Model file for the job. Use its own axes, mm. A direction names the side the tool comes from. Give positions to 0.01 mm unless a question says otherwise; leave off trailing zeros. Order: outer loops, then holes, each group sorted by start corner. A loop starts at its lowest first (then second) coordinate and runs counter-clockwise, first axis right, second up. Notation, with made-up numbers: M 35,-6.75 L 64,-6.75 A27 cw 64,30.25 Z; hole C 86.5,80.5 d1. An arc over 180 degrees is marked long. Return JSON: item names as keys, results as strings. Group by question number.
1. 3-axis set-ups, long thin cutter, end or side, ignore diameter. For faces 1 (the face through (38, 56, 3)), 2 (the face through (25.03, 56.1, 2.54)): which of +Z, -Z, +X, -X, +Y, -Y reach the whole face in a straight line?
2. Slice it at A-A on x = 29. List the corners of the cut face in (y, z), then the cut area to 3 significant figures.
3. Wall check: probe 1 along Y at (x, z) = (59, 1.3); probe 2 along Y at (x, z) = (9, 3); probe 3 along Y at (x, z) = (26, 0.9). Give the ranges that are in metal, low to high. Write a range as [from, to].
4. Pin check, flat tips, straight feed: pin 1 (1 mm diameter, centred on x = 39, z = 2, fed in from +Y); pin 2 (1 mm diameter, centred on y = 39, z = 2, fed in from +X); pin 3 (8 mm diameter, centred on x = 59.14, y = 29, fed in from -Z); pin 4 (2 mm diameter, centred on y = 56, z = 2, fed in from +X). Stop position of each tip, or through.
5. Slice it at D-D on z = 3.2. List the corners of the cut face in (x, y).
6. Slice it at B-B on x = 61.5. List the corners of the cut face in (y, z), then the cut area to 3 significant figures.
from build123d import *

# Parameters (mm, degrees)
BOSS_EXTRU_1_DEPTH      = 5
ESQUISSE3_W             = 38
ESQUISSE3_H             = 14
ESQUISSE3_W_2           = 14
ESQUISSE3_H_2           = 38
BOSS_EXTRU_2_DEPTH      = 5
ESQUISSE4_R             = 5
ESQUISSE4_R_2           = 3.5
ENL_V_MAT_EXTRU_2_DEPTH = 97.497156926
CONG_1_R                = 10


with BuildPart() as part:
    # Esquisse1 → Boss.-Extru.1 (new body)
    with BuildSketch(Plane.XY):
        Polygon((0, 0), (54.142135624, 0), (54.142135624, 40), (40, 54.142135624), (0, 54.142135624), align=None)
    extrude(amount=BOSS_EXTRU_1_DEPTH)

    # Esquisse3 → Boss.-Extru.2 (add)
    with BuildSketch(Plane.XY.offset(5)):
        with Locations((19, 61.142135624)):
            Rectangle(ESQUISSE3_W, ESQUISSE3_H)
        with Locations((61.142135624, 19)):
            Rectangle(ESQUISSE3_W_2, ESQUISSE3_H_2)
    extrude(amount=-BOSS_EXTRU_2_DEPTH)

    # Esquisse4 → Enlèv. mat.-Extru.2 (cut, through all)
    with BuildSketch(Plane.XY.offset(5)):
        with Locations((29, 59.142135624)):
            Circle(ESQUISSE4_R)
        with Locations(Location((9, 59.142135624, 0), (0, 0, 180))):
            Circle(ESQUISSE4_R)
        with Locations((59.142135624, 9)):
            Circle(ESQUISSE4_R)
        with Locations(Location((59.142135624, 29, 0), (0, 0, 180))):
            Circle(ESQUISSE4_R)
        with Locations((9.899494937, 9.899494937)):
            Circle(ESQUISSE4_R_2)
    extrude(amount=-ENL_V_MAT_EXTRU_2_DEPTH, mode=Mode.SUBTRACT)

    # Congé1
    cong_1_edges = [part.edges().sort_by_distance(p)[0] for p in [
        (0, 68.142135624, 2.5),
        (38, 68.142135624, 2.5),
        (68.142135624, 38, 2.5),
        (68.142135624, 0, 2.5),
        (0, 0, 2.5),
    ]]
    fillet(cong_1_edges, radius=CONG_1_R)


solid = part.part
Result:
{
 "1": {"face 1": "+Z, -Z, +X, +Y", "face 2": "+Z, -Z"},
 "2": {"outline": "M 0,0 L 54.14,0 L 54.14,5 L 0,5 Z; M 64.14,0 L 68.09,0 L 68.09,5 L 64.14,5 Z", "area": "290 mm2"},
 "3": {"probe 1": "y = [0.04, 4], [14, 24], [34, 37.96]", "probe 2": "y = [0.05, 6.52], [13.28, 54.14], [64.14, 68.09]", "probe 3": "y = [0, 55.14], [63.14, 68.14]"},
 "4": {"pin 1": "stops at y = 54.14", "pin 2": "stops at x = 54.14", "pin 3": "passes through", "pin 4": "stops at x = 38"},
 "5": {"outline": "M 0,10 A10 ccw 10,0 L 58.14,0 A10 ccw 68.14,10 L 68.14,28 A10 ccw 58.14,38 L 54.14,38 L 54.14,40 L 40,54.14 L 38,54.14 L 38,58.14 A10 ccw 28,68.14 L 10,68.14 A10 ccw 0,58.14 Z; hole C 9,59.14 d10; hole C 9.9,9.9 d7; hole C 29,59.14 d10; hole C 59.14,9 d10; hole C 59.14,29 d10"},
 "6": {"outline": "M 0.58,0 L 4.59,0 L 4.59,5 L 0.58,5 Z; M 13.41,0 L 24.59,0 L 24.59,5 L 13.41,5 Z; M 33.41,0 L 37.42,0 L 37.42,5 L 33.41,5 Z", "area": "96.0 mm2"}
}
